```python
from build123d import *

# Parameters (mm, degrees)
SKETCH1_R            = 85
BOSS_EXTRUDE1_DEPTH  = 150
BOSS_EXTRUDE1_DRAFT  = 5
CUT_SWEEP1_PROFILE_R = 2
SKETCH11_R           = 55
CUT_EXTRUDE1_DEPTH   = 150
CUT_EXTRUDE1_DRAFT   = 5
BOSS_EXTRUDE2_START  = -10
SKETCH13_W           = 140
SKETCH13_H           = 110
BOSS_EXTRUDE2_DEPTH  = 10
SKETCH14_R           = 10
CUT_EXTRUDE2_DEPTH   = 10
FILLET3_R            = 20
SKETCH15_R           = 3.5
CUT_EXTRUDE3_DEPTH   = 10
SKETCH17_R           = 5
BOSS_EXTRUDE3_DEPTH  = 5
CIRPATTERN1_COUNT    = 4


with BuildPart() as part:
    # Sketch1 → Boss-Extrude1 (with draft: the straight prism first)
    with BuildSketch(Plane(origin=(0, 0, 0), x_dir=(1, 0, 0), z_dir=(0, 1, 0))):
        Circle(SKETCH1_R)
    extrude(amount=-BOSS_EXTRUDE1_DEPTH)
    # Boss-Extrude1: the draft: its side faces are tilted about the plane it starts from
    boss_extrude1_sides = [part.faces().sort_by_distance(p)[0] for p in [
        (-85, -75, 0),
    ]]
    draft(boss_extrude1_sides, Plane(origin=(0, 0, 0), x_dir=(1, 0, 0), z_dir=(0, 1, 0)), BOSS_EXTRUDE1_DRAFT)

    # Cut-Sweep1: sweep along a path in Sketch2
    with BuildLine(Plane(origin=(0, 0, 0), x_dir=(1, 0, 0), z_dir=(0, 1, 0))) as cut_sweep1_path:
        CenterArc((0, 0), 65, 0, 360)
    # Cut-Sweep1 profile (on start of the path) → Cut-Sweep1 (sweep, cut)
    with BuildSketch(Plane(origin=(65, 0, 0), x_dir=(-1, 0, 0), z_dir=(0, 0, -1))):
        Circle(CUT_SWEEP1_PROFILE_R)
    sweep(path=cut_sweep1_path.line, mode=Mode.SUBTRACT)


with BuildPart() as cut_extrude1_tool:
    # Sketch11 → Cut-Extrude1 (with draft: the straight prism first)
    with BuildSketch(Plane(origin=(0, 0, 0), x_dir=(1, 0, 0), z_dir=(0, 1, 0))):
        Circle(SKETCH11_R)
    extrude(amount=-CUT_EXTRUDE1_DEPTH)
    # Cut-Extrude1: the draft: its side faces are tilted about the plane it starts from
    cut_extrude1_sides = [cut_extrude1_tool.faces().sort_by_distance(p)[0] for p in [
        (-55, -75, 0),
    ]]
    draft(cut_extrude1_sides, Plane(origin=(0, 0, 0), x_dir=(1, 0, 0), z_dir=(0, 1, 0)), CUT_EXTRUDE1_DRAFT)


with BuildPart() as part_1:
    add(part.part)

    # Cut-Extrude1: cut by cut_extrude1_tool
    add(cut_extrude1_tool.part, mode=Mode.SUBTRACT)

    # Sketch13 → Boss-Extrude2 (add)
    with BuildSketch(Plane(origin=(0, 0, 0), x_dir=(1, 0, 0), z_dir=(0, 1, 0)).offset(BOSS_EXTRUDE2_START)):
        with Locations((-130.53, 0)):
            Rectangle(SKETCH13_W, SKETCH13_H)
    extrude(amount=-BOSS_EXTRUDE2_DEPTH)

    # Sketch14 → Cut-Extrude2 (cut)
    with BuildSketch(Plane(origin=(0, -10, 0), x_dir=(1, 0, 0), z_dir=(0, 1, 0))):
        with Locations(Location((-150.53, 0, 0), (0, 0, 270))):
            Circle(SKETCH14_R)
    extrude(amount=-CUT_EXTRUDE2_DEPTH, mode=Mode.SUBTRACT)

    # Fillet3
    fillet3_edges = [part_1.edges().sort_by_distance(p)[0] for p in [
        (-200.53, -15, 55),
        (-200.53, -15, -55),
    ]]
    fillet(fillet3_edges, radius=FILLET3_R)

    # Sketch15 → Cut-Extrude3 (cut)
    with BuildSketch(Plane(origin=(0, -10, 0), x_dir=(1, 0, 0), z_dir=(0, 1, 0))):
        with Locations(Location((-185.53, 35, 0), (0, 0, 270))):
            Circle(SKETCH15_R)
        with Locations(Location((-115.53, 35, 0), (0, 0, 270))):
            Circle(SKETCH15_R)
        with Locations(Location((-115.53, -35, 0), (0, 0, 270))):
            Circle(SKETCH15_R)
        with Locations(Location((-185.53, -35, 0), (0, 0, 270))):
            Circle(SKETCH15_R)
    extrude(amount=-CUT_EXTRUDE3_DEPTH, mode=Mode.SUBTRACT)

    # Sketch17 → Boss-Extrude3 (add)
    with BuildSketch(Plane.XZ.offset(150)):
        with BuildLine():
            Line((-10, 136.694847673), (10, 136.694847673))
            ThreePointArc((10, 136.694847673), (17.071067812, 133.765915485), (20, 126.694847673))
            Line((20, 126.694847673), (20, 82.304982624))
            Line((20, 82.304982624), (-20, 82.304982624))
            Line((-20, 82.304982624), (-20, 126.694847673))
            ThreePointArc((-20, 126.694847673), (-17.071067812, 133.765915485), (-10, 136.694847673))
        make_face()
        with Locations(Location((0, 120, 0), (0, 0, 270))):
            Circle(SKETCH17_R, mode=Mode.SUBTRACT)
    boss_extrude3 = extrude(amount=-BOSS_EXTRUDE3_DEPTH)

    # CirPattern1: Boss-Extrude3 ×4 about axis
    cirpattern1_axis = Axis((0, 0, 0), (0, 1, 0))
    for i in range(1, CIRPATTERN1_COUNT):
        add(boss_extrude3.rotate(cirpattern1_axis, i * 360 / CIRPATTERN1_COUNT))


solid = part_1.part
```
Geometry: final body of the model. Coordinates: model frame, mm. A direction names the side the tool comes from. Coordinates: 2 decimals unless noted, no trailing zeros. Order: outer loops, then holes, each group sorted by start corner. A loop starts at its lowest first (then second) coordinate and runs counter-clockwise, first axis right, second up. Notation, with made-up numbers: M 86,-29 L 97,-29 A19 ccw 97,0 Z; hole C 11,-31 d9. An arc over 180 degrees is marked long. Answer in a Markdown table with one row per item. Add a question column.
Q1. Section query B-B on z = 120. Return the cut outline in (x, y), and give its area (3 significant figures).
Q2. Section query D-D on y = -88. Return the cut outline in (x, z).
Q3. Section query C-C on y = -107. Return the cut outline in (x, z), and give its area (3 significant figures).
Q4. Contact query for flat-ended pins moving along their axis: P1, Ø1.5, axis at x = 8, y = -127.5, coming from the +Z side; P2, Ø4, axis at x = -106.5, y = -146.5, coming from the -Z side; P3, Ø2.5, axis at y = -147, z = -110.5, coming from the -X side. Output: stop coordinate, or through.
Q5. Section query A-A on x = 120. Return the cut outline in (y, z).
Q6. Mould query, pull axis X, two halves, no side actions, for faces 3 (the cylindrical face through (115.381, -147.535, 1.915)), 4 (the cylindrical face through (-133.843, -147.535, 16.993)), 5 (the cylindrical face through (16.993, -147.535, 133.843)), 6 (the conical face through (-11.91, -73.95, -90.69)). Classes: released by +X, released by -X, zero draft, split by the parting line, or undercut.
Q7. Reachability of faces 1 (the cylindrical face through (-115.381, -147.535, -1.915)), 2 (the flat face through (-61, -150, 31)) from +Z, -Z, +X, -X, +Y, -Y: full face, straight path, thin tool, end or side. Return the list, or none.
Q8. Line query: L1, parallel to Z at x = -115, y = -17; L2, parallel to Z at x = -120, y = -147.05; L3, parallel to X at y = -12.5, z = 35.5. Output: solid intervals per line, ascending.
Completed:
| question | item | result |
|---|---|---|
| 1 | outline | M -20,-150 L -5,-150 L -5,-145 L -20,-145 Z; M 5,-150 L 20,-150 L 20,-145 L 5,-145 Z |
| 1 | area | 150 mm2 |
| 2 | outline | C 0,0 d185.4; hole C 0,0 d125.4 |
| 3 | outline | C 0,0 d188.72; hole C 0,0 d128.72 |
| 3 | area | 15,000 mm2 |
| 4 | P1 | stops at z = 95.91 |
| 4 | P2 | stops at z = -20 |
| 4 | P3 | stops at x = -20 |
| 5 | outline | M -150,-20 L -145,-20 L -145,-5 L -150,-5 Z; M -150,5 L -145,5 L -145,20 L -150,20 Z |
| 6 | face 3 | undercut |
| 6 | face 4 | released by -X |
| 6 | face 5 | released by +X |
| 6 | face 6 | split by the parting line |
| 7 | face 1 | -Y |
| 7 | face 2 | +Z, -Z, +X, -X, -Y |
| 8 | L1 | z = -55 to -38.46, -31.54 to 31.54, 38.46 to 55 |
| 8 | L2 | z = -20 to -5, 5 to 20 |
| 8 | L3 | x = -200.52 to -188.99, -182.07 to -118.99, -112.07 to -43.43, 43.43 to 78.43 |
